from build123d import *

# Parameters (mm, degrees)
SKETCH1_R           = 6
SKETCH1_R_2         = 5.05
BOSS_EXTRUDE1_DEPTH = 3.5
SKETCH4_R           = 6
BOSS_EXTRUDE2_DEPTH = 0.5
SKETCH5_W           = 3
SKETCH5_H           = 1.177915389
CUT_EXTRUDE3_DEPTH  = 2.5
CUT_EXTRUDE4_DEPTH  = 1.5
FILLET1_R           = 0.5


with BuildPart() as part:
    # Sketch1 → Boss-Extrude1 (new body)
    with BuildSketch(Plane(origin=(0, 0, 0), x_dir=(1, 0, 0), z_dir=(0, 1, 0))):
        Circle(SKETCH1_R)
        Circle(SKETCH1_R_2, mode=Mode.SUBTRACT)
    extrude(amount=BOSS_EXTRUDE1_DEPTH)

    # Sketch4 → Boss-Extrude2 (add)
    with BuildSketch(Plane.XZ):
        Circle(SKETCH4_R)
    extrude(amount=BOSS_EXTRUDE2_DEPTH)

    # Sketch5 → Cut-Extrude3 (cut)
    with BuildSketch(Plane.XZ.offset(-3.5)):
        with Locations((0, 5.411042306)):
            Rectangle(SKETCH5_W, SKETCH5_H)
    extrude(amount=CUT_EXTRUDE3_DEPTH, mode=Mode.SUBTRACT)

    # Sketch7 → Cut-Extrude4 (cut, through all)
    with BuildSketch(Plane(origin=(0, 0, 0), x_dir=(1, 0, 0), z_dir=(0, 1, 0))):
        with BuildLine():
            Line((4.062326919, -3), (-4.062326919, -3))
            ThreePointArc((-4.062326919, -3), (0, -5.05), (4.062326919, -3))
        make_face()
        with BuildLine():
            Line((4.062326919, 3), (-4.062326919, 3))
            ThreePointArc((-4.062326919, 3), (0, 5.05), (4.062326919, 3))
        make_face()
    extrude(amount=-CUT_EXTRUDE4_DEPTH, mode=Mode.SUBTRACT)

    # Fillet1
    fillet1_edges = [part.edges().sort_by_distance(p)[0] for p in [
        (-3.674234614, 3.5, -4.74341649),
        (-1.5, 1, 5.315779815),
        (1.5, 1, 5.315779815),
    ]]
    fillet(fillet1_edges, radius=FILLET1_R)


solid = part.part
Input: part model. Units: mm. Frame: model coordinates. A direction names the side the tool comes from. Round coordinates to 2 decimals unless told otherwise and drop trailing zeros. Order: outer loops, then holes, each group sorted by start corner. A loop starts at its lowest first (then second) coordinate and runs counter-clockwise, first axis right, second up. Notation, with made-up numbers: (78, 7.25) - (104, 7.25) arc R21 ccw to (104, 42.25) - close; hole circle Ø10 at (-33, 49.5). An arc over 180 degrees is marked (long way). Use a Markdown table: item, result.
1. Material intervals for probe 1 along Z at (x, y) = (0, 0.9); probe 2 along X at (y, z) = (3.15, 2.5), sorted ascending.
Evaluation:
| item | result |
|---|---|
| probe 1 | -6 to -5.05, 5.05 to 6 |
| probe 2 | -5.43 to -4.39, 4.39 to 5.43 |
2. Mould query, pull axis Z, two halves, no side actions, for faces 1 (the face through (0, 0, 0)), 2 (the face through (-1.5, 3, 5)), 3 (the face through (-1.301, 1.274, -5.857)). Classes: +Z half, -Z half, draft (parallel to the pull), parting line (faces both ways), or undercut.
Evaluation:
| item | result |
|---|---|
| face 1 | undercut |
| face 2 | draft |
| face 3 | parting line |
3. First-contact query: pin 1 (5 mm diameter, centred on x = -1, z = 0, fed in from +Y); pin 2 (1.1 mm diameter, centred on y = 3, z = 5.5, fed in from -X); pin 3 (1.5 mm diameter, centred on y = 1, z = 1, fed in from +X). Flat tips, straight axial feed; report the tip coordinate or a pass-through.
Evaluation:
| item | result |
|---|---|
| pin 1 | y = 0 |
| pin 2 | x = -3.39 |
| pin 3 | x = 5.99 |
4. Section A-A on x = 0. Return the cut outline in (y, z), then the cut area to 3 significant figures.
Evaluation:
| item | result |
|---|---|
| outline | (-0.5, -6) - (3, -6) arc R0.5 ccw to (3.5, -5.5) - (3.5, -5.05) - (-0.5, -5.05) - close; (-0.5, -3) - (0, -3) - (0, 3) - (-0.5, 3) - close; (-0.5, 5.05) - (1, 5.05) - (1, 6) - (-0.5, 6) - close |
| area | 8.17 mm^2 |
5. Access query for faces 4 (the face through (0, -0.5, 0)), 5 (the face through (1.5, 3, 5)). Directions: +Z, -Z, +X, -X, +Y, -Y. A direction counts if a zero-diameter tool reaches every point of the face in a straight line with its end or side. Return the directions, or none.
Evaluation:
| item | result |
|---|---|
| face 4 | +Z, -Z, +X, -X, -Y |
| face 5 | +Z, +Y |
6. Section D-D on y = 2.75. Return the cut outline in (x, z).
Evaluation:
| item | result |
|---|---|
| outline | (-1.5, 4.82) - (-1.5, 5.81) arc R6 ccw (long way) to (1.5, 5.81) - (1.5, 4.82) arc R5.05 cw (long way) to start |
7. Section B-B on z = 0. Return the cut outline in (x, y).
Evaluation:
| item | result |
|---|---|
| outline | (-6, -0.5) - (6, -0.5) - (6, 3) arc R0.5 ccw to (5.5, 3.5) - (5.05, 3.5) - (5.05, 0) - (-5.05, 0) - (-5.05, 3.5) - (-5.5, 3.5) arc R0.5 ccw to (-6, 3) - close |
8. Section C-C on y = 0.5. Return the cut outline in (x, z).
Evaluation:
| item | result |
|---|---|
| outline | circle Ø12 at (0, 0); hole circle Ø10.1 at (0, 0) |
